Read the model definition and answer for the solid it produces. Units are mm, in the model's axes. Face numbers are marked on the shaded views. Coordinates: 2 decimals unless noted, no trailing zeros. Order: outer loops, then holes, each group sorted by start corner. A loop starts at its lowest first (then second) coordinate and runs counter-clockwise, first axis right, second up. Notation, with made-up numbers: (11, 72.5) -> (21, 72.5) arc R16 cw to (21, 95.5) -> close; hole circle Ø8 at (79, -16.5). An arc over 180 degrees is marked (long way). Answer as a JSON object with one key per item and string values. Group by question number.
1) Section C-C on x = 36 is taken. Determine the outline of the cut face in (y, z).
2) Consider L1, parallel to Z at x = 12, y = 6.75; L2, parallel to Z at x = 36, y = 0.95; L3, parallel to Z at x = 7, y = 3.75. Determine where each line is inside the solid, lowest interval first.
3) Given pin 1 (4.5 mm diameter, centred on y = 5, z = -47.5, fed in from +X); pin 2 (5 mm diameter, centred on x = 14, z = -13, fed in from +Y); pin 3 (1.2 mm diameter, centred on y = 5, z = -14.5, fed in from -X), each flat-ended and moving along its own axis, determine where each tip first touches the part or whether it passes through.
4) Section B-B on z = -13 is taken. Count the separate pieces of the cut face and the enclosed holes in it, and give its area (3 significant figures).
5) Section D-D on z = -6 is taken. Determine the outline of the cut face in (x, y), and give its area (3 significant figures).
6) Section A-A on x = 7 is taken. Determine the outline of the cut face in (y, z).
7) Determine the mould class of the marked faces 1, 2 and 3 for opening direction Z: released by +Z, released by -Z, zero draft, split by the parting line, or undercut.
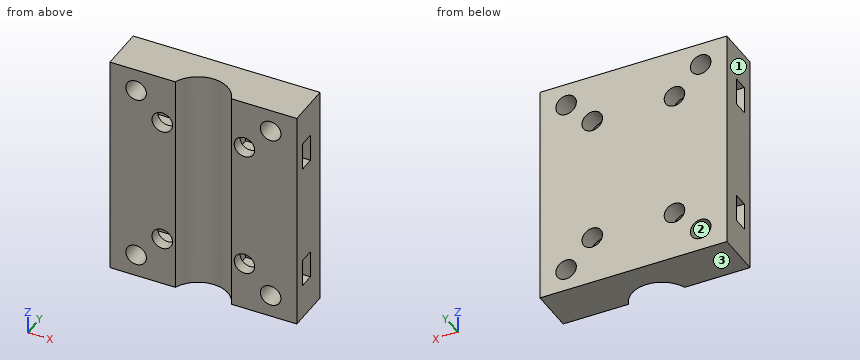
from build123d import *

# Parameters (mm, degrees)
SKETCH1_W                      = 50
SKETCH1_H                      = 60
BOSS_EXTRUDE1_DEPTH            = 12
CUT_EXTRUDE1_DEPTH             = 80.018985061
F_5_5_5_5_DIAMETER_HOLE1_D     = 5.5
F_5_5_5_5_DIAMETER_HOLE1_DEPTH = 30
F_5_5_5_5_DIAMETER_HOLE1_TIP   = 1.652366702
SKETCH5_W                      = 7.3
SKETCH5_H                      = 4
CUT_EXTRUDE2_DEPTH             = 17.3
SKETCH6_W                      = 7.3
SKETCH6_H                      = 4
CUT_EXTRUDE3_DEPTH             = 17.3
F_5_5_5_5_DIAMETER_HOLE2_D     = 5.5


with BuildPart() as part:
    # Sketch1 → Boss-Extrude1 (new body)
    with BuildSketch(Plane(origin=(0, 0, 0), x_dir=(1, 0, 0), z_dir=(0, 1, 0))):
        with Locations((25, 30)):
            Rectangle(SKETCH1_W, SKETCH1_H)
    extrude(amount=BOSS_EXTRUDE1_DEPTH)

    # Sketch2 → Cut-Extrude1 (cut, through all)
    with BuildSketch(Plane.XY):
        with BuildLine():
            Line((17.5, 0), (32.5, 0))
            ThreePointArc((32.5, 0), (25, 5.216117819), (17.5, 0))
        make_face()
    extrude(amount=-CUT_EXTRUDE1_DEPTH, mode=Mode.SUBTRACT)

    # Ø5.5 (5.5) Diameter Hole1
    with Locations(Plane.XZ):
        with Locations((14, -13), (36, -13), (14, -47), (36, -47)):
            Hole(F_5_5_5_5_DIAMETER_HOLE1_D / 2, depth=F_5_5_5_5_DIAMETER_HOLE1_DEPTH)
            with Locations((0, 0, -(F_5_5_5_5_DIAMETER_HOLE1_DEPTH + F_5_5_5_5_DIAMETER_HOLE1_TIP / 2))):  # 118° drill point
                Cone(0, F_5_5_5_5_DIAMETER_HOLE1_D / 2, F_5_5_5_5_DIAMETER_HOLE1_TIP, mode=Mode.SUBTRACT)

    # Sketch5 → Cut-Extrude2 (cut)
    with BuildSketch(Plane.ZY):
        with Locations((-47, 5)):
            Rectangle(SKETCH5_W, SKETCH5_H)
        with Locations((-13, 5)):
            Rectangle(SKETCH5_W, SKETCH5_H)
    extrude(amount=-CUT_EXTRUDE2_DEPTH, mode=Mode.SUBTRACT)

    # Sketch6 → Cut-Extrude3 (cut)
    with BuildSketch(Plane(origin=(50, 0, 0), x_dir=(0, 0, -1), z_dir=(1, 0, 0))):
        with Locations((13, 5)):
            Rectangle(SKETCH6_W, SKETCH6_H)
        with Locations((47, 5)):
            Rectangle(SKETCH6_W, SKETCH6_H)
    extrude(amount=-CUT_EXTRUDE3_DEPTH, mode=Mode.SUBTRACT)

    # Ø5.5 (5.5) Diameter Hole2 (through all)
    with Locations(Plane(origin=(0, 12, 0), x_dir=(-1, 0, 0), z_dir=(0, 1, 0))):
        with Locations((-43, -6), (-7, -6), (-7, -54), (-43, -54)):
            Hole(F_5_5_5_5_DIAMETER_HOLE2_D / 2)


solid = part.part
Worked answers:
{
 "1": {"outline": "(0, -60) -> (12, -60) -> (12, -49.75) -> (7, -49.75) -> (7, -50.65) -> (3, -50.65) -> (3, -49.75) -> (0, -49.75) -> close; (0, -44.25) -> (3, -44.25) -> (3, -43.35) -> (7, -43.35) -> (7, -44.25) -> (12, -44.25) -> (12, -15.75) -> (7, -15.75) -> (7, -16.65) -> (3, -16.65) -> (3, -15.75) -> (0, -15.75) -> close; (0, -10.25) -> (3, -10.25) -> (3, -9.35) -> (7, -9.35) -> (7, -10.25) -> (12, -10.25) -> (12, 0) -> (0, 0) -> close"},
 "2": {"L1": "z = -60 to -50.65, -43.35 to -16.65, -9.35 to 0", "L2": "z = -60 to -49.75, -44.25 to -15.75, -10.25 to 0", "L3": "z = -60 to -56.75, -51.25 to -50.65, -43.35 to -16.65, -9.35 to -8.75, -3.25 to 0"},
 "3": {"pin 1": "stops at x = 50", "pin 2": "passes through", "pin 3": "stops at x = 17.3"},
 "4": {"separate pieces": "5", "enclosed holes": "0", "area": "317 mm²"},
 "5": {"outline": "(0, 0) -> (4.25, 0) -> (4.25, 12) -> (0, 12) -> close; (9.75, 0) -> (17.5, 0) arc R8 cw to (32.5, 0) -> (40.25, 0) -> (40.25, 12) -> (9.75, 12) -> close; (45.75, 0) -> (50, 0) -> (50, 12) -> (45.75, 12) -> close", "area": "411 mm²"},
 "6": {"outline": "(0, -60) -> (12, -60) -> (12, -56.75) -> (0, -56.75) -> close; (0, -51.25) -> (12, -51.25) -> (12, -8.75) -> (0, -8.75) -> close; (0, -3.25) -> (12, -3.25) -> (12, 0) -> (0, 0) -> close; hole (3, -50.65) -> (7, -50.65) -> (7, -43.35) -> (3, -43.35) -> close; hole (3, -16.65) -> (7, -16.65) -> (7, -9.35) -> (3, -9.35) -> close"},
 "7": {"face 1": "zero draft", "face 2": "undercut", "face 3": "released by -Z"}
}
